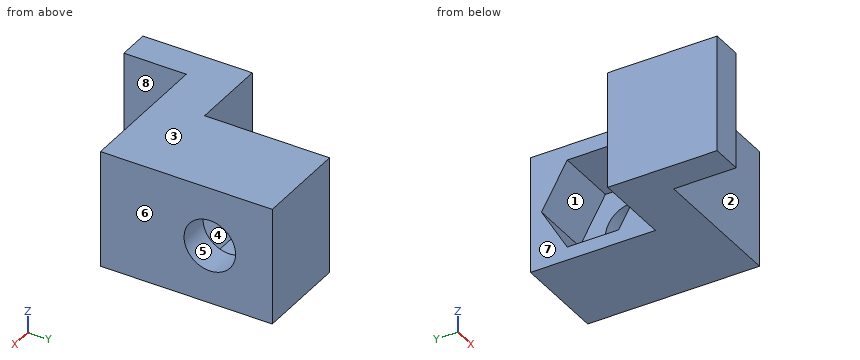
Autodesk Inventor part; units mm, degrees
ref_plane "YZ Plane" through (0, 0, 0) normal (1, 0, 0) x (0, 1, 0)
ref_plane "XZ Plane" through (0, 0, 0) normal (0, 1, 0) x (-1, 0, 0)
ref_plane "XY Plane" through (0, 0, 0) normal (0, 0, 1) x (1, 0, 0)
sketch "Sketch1" plane through (0, 0, 0) normal (0, 0, 1) x (1, 0, 0)
  line L0 (31.7273, 1.5) -> (12.134, 1.5)
  line L1 (31.7273, -1.5) -> (12.134, -1.5)
  line L2 (16.2594, -4) -> (22.2594, -4)
  line L3 (22.2594, -4) -> (22.2594, 4)
  line L4 (22.2594, 4) -> (16.2594, 4)
  line L5 (16.2594, 4) -> (16.2594, -4)
  line L6 (16.2594, -4) -> (22.2594, 4) construction
  line L7 (22.2594, -4) -> (16.2594, 4) construction
  point P0 (0, 0)
  point P1 (19.2594, 0)
  dimension "d0" = 8
  dimension "d1" = 6
extrude "Extrusion1" add sketch "Sketch1" along normal mid plane 7.5
sketch "Sketch2" plane through (16.2594, -4, 3.75) normal (-1, 0, 0) x (0, 0, 1)
  line L0 (0, 0) -> (-7.5, 0)
  line L1 (0, 8) -> (0, 0)
  line L2 (-7.5, 8) -> (0, 8)
  line L3 (-7.5, 0) -> (-7.5, 8)
  circle A0 centre (-3.75, 4) radius 1.65
  dimension "d17" = 3.3
extrude "Extrusion2" cut sketch "Sketch2" against normal through all contours A0
sketch "Sketch3" plane through (16.2594, -4, 3.75) normal (-1, 0, 0) x (0, 0, 1)
  point P0 (-3.75, 4)
sketch "Sketch4" plane through (16.2594, -4, 3.75) normal (-1, 0, 0) x (0, 0, 1)
  line L0 (-0.953, 2.3546) -> (-3.803, 0.7091)
  line L1 (-3.803, 0.7091) -> (-6.653, 2.3546)
  line L2 (-6.653, 2.3546) -> (-6.653, 5.6454)
  line L3 (-6.653, 5.6454) -> (-3.803, 7.2909)
  line L4 (-3.803, 7.2909) -> (-0.953, 5.6454)
  line L5 (-0.953, 5.6454) -> (-0.953, 2.3546)
  line L6 (-7.5, 0) -> (-7.5, 8)
  point P0 (-3.803, 4)
  dimension "d18" = 5.7
extrude "Extrusion3" cut sketch "Sketch4" against normal blind 4
sketch "Sketch5" plane through (0, 0, 3.75) normal (0, 0, 1) x (1, 0, 0)
  line L0 (16.2594, -4) -> (22.2594, -4)
  line L1 (22.2594, -4) -> (22.2594, 4)
  line L2 (22.2594, 4) -> (16.2594, 4)
  line L3 (16.2594, 4) -> (16.2594, -4)
  line L4 (16.2594, -4) -> (22.2594, -4)
  line L5 (22.2594, -4) -> (11.2594, -4)
  line L6 (11.2594, -4) -> (11.2594, -7)
  line L7 (11.2594, -7) -> (22.2594, -7)
  line L8 (22.2594, -7) -> (22.2594, -4)
  line L9 (11.2594, -7) -> (13.2594, -7)
  line L10 (13.2594, -7) -> (13.2594, -11)
  line L11 (13.2594, -11) -> (11.2594, -11)
  line L12 (11.2594, -11) -> (11.2594, -7)
  point P0 (0, 0)
  dimension "d13" = 11
  dimension "d14" = 3
  dimension "d15" = 2
  dimension "d16" = 4
extrude "Extrusion4" add sketch "Sketch5" against normal up to surface (7.5 mm away) contours L0 L8 L7 L6 L5 | L7 L10 L11 L12
properties part number "TMP_Holder_MTP"
Input: part model. Units: mm. Frame: model coordinates. Face numbers are marked on the shaded views. A direction names the side the tool comes from. Round coordinates to 2 decimals unless told otherwise and drop trailing zeros. Loops run counter-clockwise (first coordinate to the right, second up) from the corner with the lowest first, then second, coordinate; pieces in that order, holes last. Notation, with made-up numbers: (70.25, 30.25) -> (97.25, 30.25) arc R21 cw to (97.25, 56.25) -> close; hole circle Ø6 at (23, -5). An arc over 180 degrees is marked (long way). Use one line per item in the form item = value. Start each with the question number.
Item 1: Section query C-C on y = -1. Return the cut outline in (x, z), then the cut area to 3 significant figures.
Item 2: Set-up query: the marked faces 4, 5, 6, 7 and 8. Return all of +Z, -Z, +X, -X, +Y, -Y with unobstructed straight access to the full face (end or side cutting, diameter ignored); none if empty.
Item 3: Mould query, pull axis Z, two halves, no side actions, for the marked faces 1, 2 and 3. Classes: pulls with the +Z half, pulls with the -Z half, needs draft (parallel to the pull), parting line crosses it, or undercut.
Item 4: Section query D-D on y = -2.5. Return the cut outline in (x, z).
Item 5: Section query A-A on x = 18.25. Return the cut outline in (y, z).
Item 6: Contact query for flat-ended pins moving along their axis: pin 1 Ø4.5 at (y, z) = (-10, -1) entering from +X; pin 2 Ø1.5 at (x, z) = (13.5, 0) entering from +Y; pin 3 Ø4.5 at (y, z) = (0, 0) entering from -X. Output: stop coordinate, or through.
Item 7: Section query B-B on z = -0.25. Return the cut outline in (x, y), then the cut area to 3 significant figures.
Item 8: Material intervals for L1, parallel to Y at x = 21.5, z = 0; L2, parallel to X at y = 0.25, z = -1.75; L3, parallel to Y at x = 12, z = 1.5, sorted ascending. Write a range as from..to.
Ans:
q1.outline = (16.26, -3.75) -> (22.26, -3.75) -> (22.26, -1.31) -> (20.26, -1.31) -> (20.26, -2.9) -> (16.26, -2.9) -> close; (16.26, 2.8) -> (20.26, 2.8) -> (20.26, 1.31) -> (22.26, 1.31) -> (22.26, 3.75) -> (16.26, 3.75) -> close
q1.area = 17.0 mm^2
q2.face_4 = -X
q2.face_5 = +X, -X
q2.face_6 = +Z, -Z, +X, +Y, -Y
q2.face_7 = +Z, -Z, -X, +Y
q2.face_8 = +Z, -Z, +X, -Y
q3.face_1 = undercut
q3.face_2 = needs draft
q3.face_3 = pulls with the +Z half
q4.outline = (16.26, -3.75) -> (22.26, -3.75) -> (22.26, 3.75) -> (16.26, 3.75) -> (16.26, 1.32) -> (20.26, 1.32) -> (20.26, -1.42) -> (16.26, -1.42) -> close
q5.outline = (-7, -3.75) -> (4, -3.75) -> (4, 3.75) -> (-7, 3.75) -> close; hole (-3.29, -0.05) -> (-1.65, -2.9) -> (1.65, -2.9) -> (3.29, -0.05) -> (1.65, 2.8) -> (-1.65, 2.8) -> close
q6.pin_1 = 13.26
q6.pin_2 = -4
q6.pin_3 = 20.26
q7.outline = (11.26, -11) -> (13.26, -11) -> (13.26, -7) -> (22.26, -7) -> (22.26, -1.63) -> (20.26, -1.63) -> (20.26, -3.18) -> (16.26, -3.18) -> (16.26, -4) -> (11.26, -4) -> close; (16.26, 3.18) -> (20.26, 3.18) -> (20.26, 1.63) -> (22.26, 1.63) -> (22.26, 4) -> (16.26, 4) -> close
q7.area = 57.1 mm^2
q8.L1 = -7..-1.65, 1.65..4
q8.L2 = 20.26..22.26
q8.L3 = -11..-4
